The figure shows three views and two pictorial views of one solid part (mm, origin at its lowest corner). Answer the questions. A direction names the side the tool comes from. Coordinates: 2 decimals unless noted, no trailing zeros. Write each loop counter-clockwise with the first axis right and the second up, starting at its lowest first coordinate (ties: lowest second). Pieces come first, ordered by that corner, then holes.
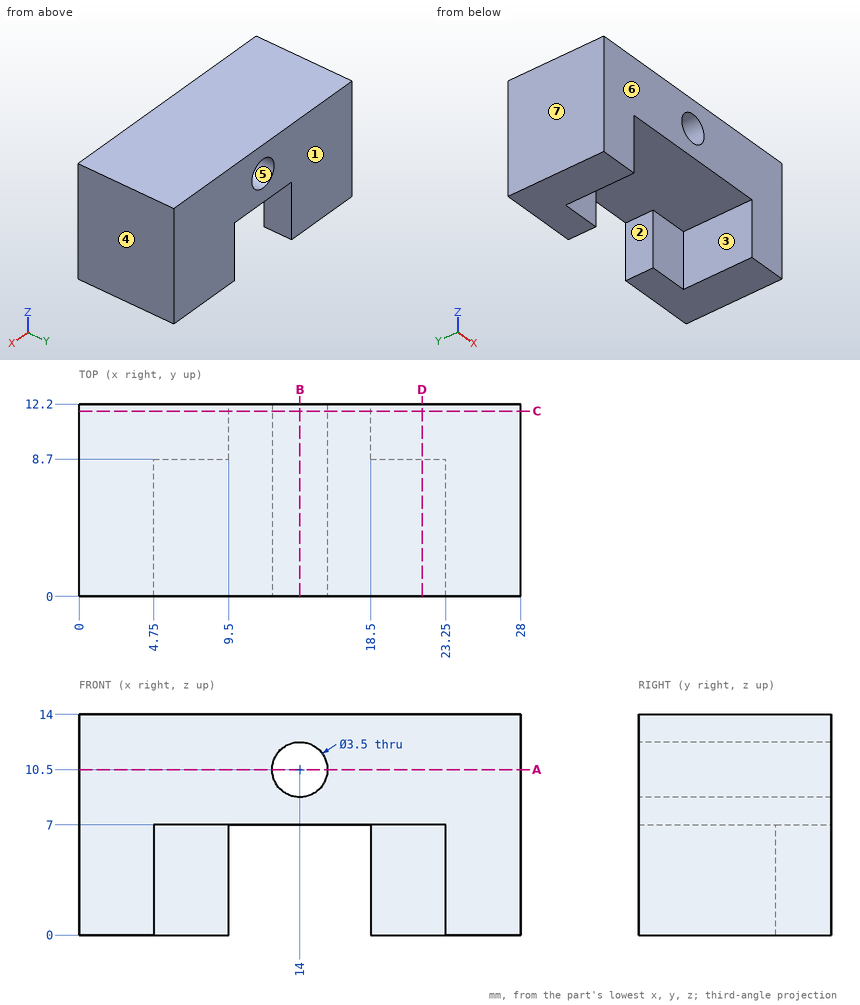
1. For a pull along X with two mould halves and no side action, classify the marked faces 4, 5, 6 and 7 as pulls with the +X half, pulls with the -X half, needs draft (parallel to the pull), parting line crosses it, or undercut.
Results found:
face 4: pulls with the +X half
face 5: undercut
face 6: needs draft
face 7: pulls with the -X half
2. Section D-D on x = 21.75 is taken. Give the vertices of the cut face in (y, z).
Results found:
outline: (0, 7) - (8.7, 7) - (8.7, 0) - (12.2, 0) - (12.2, 14) - (0, 14) - close
3. Find the intervals of material crossed by L1, parallel to Z at x = 14, y = 4.75; L2, parallel to X at y = 11.5, z = 1.25; L3, parallel to X at y = 8, z = 10.5, in increasing order.
Results found:
L1: z = 7 to 8.75, 12.25 to 14
L2: x = 0 to 9.5, 18.5 to 28
L3: x = 0 to 12.25, 15.75 to 28
4. Section B-B on x = 14 is taken. Give the vertices of the cut face in (y, z), then the cut area to 3 significant figures.
Results found:
outline: (0, 7) - (12.2, 7) - (12.2, 8.75) - (0, 8.75) - close; (0, 12.25) - (12.2, 12.25) - (12.2, 14) - (0, 14) - close
area: 42.7 mm2
5. A tool of negligible diameter and unlimited length cuts with its end or side. For the marked faces 1, 2 and 3, from which of +Z, -Z, +X, -X, +Y, -Y can it reach the whole face along a straight path? Write none if from no direction.
Results found:
face 1: +Z, -Z, +X, -X, +Y
face 2: -Z, +Y, -Y
face 3: -Z, -Y
6. Section C-C on y = 11.75 is taken. Give the vertices of the cut face in (x, z).
Results found:
outline: (0, 0) - (9.5, 0) - (9.5, 7) - (18.5, 7) - (18.5, 0) - (28, 0) - (28, 14) - (0, 14) - close; hole circle Ø3.5 at (14, 10.5)
7. Section A-A on z = 10.5 is taken. Give the vertices of the cut face in (x, y), then the cut area to 3 significant figures.
Results found:
outline: (0, 0) - (12.25, 0) - (12.25, 12.2) - (0, 12.2) - close; (15.75, 0) - (28, 0) - (28, 12.2) - (15.75, 12.2) - close
area: 299 mm2
8. A flat-ended cylindrical pin translates along its axis: P1, Ø5, axis at x = 11, y = 2.5, coming from the -Z side. Find the tip coordinate at first contact, or state that the pin passes through.
Results found:
P1: stops at z = 7
